```python
from build123d import *

# Parameters (mm, degrees)
SKETCH1_W           = 685.8
SKETCH1_H           = 165.1
BOSS_EXTRUDE1_DEPTH = 12.7
SKETCH2_R           = 3.175
CUT_EXTRUDE1_DEPTH  = 26.67
SKETCH3_R           = 3.5
CUT_EXTRUDE2_DEPTH  = 34
SKETCH4_R           = 6
CUT_EXTRUDE3_DEPTH  = 9.85
SKETCH5_R           = 1.7526
CUT_EXTRUDE4_DEPTH  = 19.05
SKETCH7_R           = 1.7526
CUT_EXTRUDE5_DEPTH  = 11.43


with BuildPart() as part:
    # Sketch1 → Boss-Extrude1 (new body)
    with BuildSketch(Plane.XY):
        Rectangle(SKETCH1_W, SKETCH1_H)
    extrude(amount=BOSS_EXTRUDE1_DEPTH)

    # Sketch2 → Cut-Extrude1 (cut)
    with BuildSketch(Plane(origin=(342.9, 0, 0), x_dir=(0, 0, -1), z_dir=(1, 0, 0))):
        with Locations((-6.35, -6.35)):
            Circle(SKETCH2_R)
    cut_extrude1 = extrude(amount=-CUT_EXTRUDE1_DEPTH, mode=Mode.SUBTRACT)

    # Sketch3 → Cut-Extrude2 (cut)
    with BuildSketch(Plane(origin=(342.9, 0, 0), x_dir=(0, 0, -1), z_dir=(1, 0, 0))):
        with Locations((-6.35, 38.1)):
            Circle(SKETCH3_R)
        with Locations(Location((-6.35, -50.8, 0), (0, 0, 180))):
            Circle(SKETCH3_R)
    cut_extrude2 = extrude(amount=-CUT_EXTRUDE2_DEPTH, mode=Mode.SUBTRACT)

    # Mirror2: Cut-Extrude1, Cut-Extrude2 across plane
    add(cut_extrude1.mirror(Plane(origin=(0, 0, 0), x_dir=(0, 0, 1), z_dir=(1, 0, 0))), mode=Mode.SUBTRACT)
    add(cut_extrude2.mirror(Plane(origin=(0, 0, 0), x_dir=(0, 0, 1), z_dir=(1, 0, 0))), mode=Mode.SUBTRACT)

    # Sketch4 → Cut-Extrude3 (cut)
    with BuildSketch(Plane.XY.offset(12.7)):
        with Locations((-308.9, 38.1)):
            Circle(SKETCH4_R)
        with Locations((308.9, -50.8)):
            Circle(SKETCH4_R)
        with Locations(Location((-308.9, -50.8, 0), (0, 0, 179.999999983))):
            Circle(SKETCH4_R)
        with Locations((308.9, 38.1)):
            Circle(SKETCH4_R)
    extrude(amount=-CUT_EXTRUDE3_DEPTH, mode=Mode.SUBTRACT)

    # Sketch5 → Cut-Extrude4 (cut)
    with BuildSketch(Plane.XZ.offset(82.55)):
        with Locations(Location((-209.55, 6.35, 0), (0, 0, 270))):
            Circle(SKETCH5_R)
        with Locations(Location((-69.85, 6.35, 0), (0, 0, 270))):
            Circle(SKETCH5_R)
        with Locations(Location((69.85, 6.35, 0), (0, 0, 270))):
            Circle(SKETCH5_R)
        with Locations(Location((209.55, 6.35, 0), (0, 0, 270))):
            Circle(SKETCH5_R)
    extrude(amount=-CUT_EXTRUDE4_DEPTH, mode=Mode.SUBTRACT)

    # Sketch7 → Cut-Extrude5 (cut)
    with BuildSketch(Plane(origin=(0, 0, 0), x_dir=(-1, 0, 0), z_dir=(0, 0, -1))):
        with Locations((278.43375, -61.9125)):
            Circle(SKETCH7_R)
        with Locations(Location((232.39625, -61.9125, 0), (0, 0, 180))):
            Circle(SKETCH7_R)
        with Locations((-232.39625, -61.9125)):
            Circle(SKETCH7_R)
        with Locations(Location((-278.43375, -61.9125, 0), (0, 0, 180))):
            Circle(SKETCH7_R)
    extrude(amount=-CUT_EXTRUDE5_DEPTH, mode=Mode.SUBTRACT)


solid = part.part
```
Could you check a few things on this model? Use its own coordinates, in mm. A direction names the side the tool comes from. Round coordinates to 2 decimals unless told otherwise and drop trailing zeros.
(1) Which directions (+Z, -Z, +X, -X, +Y, -Y) give clear straight access to the entire face, cutting with the end or side of a thin tool? Please do faces 1 (the face through (-309, -51, 2.85)), 2 (the face through (342.9, -1, 6)).
Findings below:
face 1: +Z
face 2: +Z, -Z, +X, +Y, -Y
(2) Thinking about a two-plate mould opening in Y: for faces 3 (the face through (-5, 82.55, 6)), 4 (the face through (302.906, 38.364, 7.844)), 5 (the face through (-5, -82.55, 6)), 6 (the face through (-5, 1, 0)), which applies, +Y half, -Y half, draft (parallel to the pull), parting line (faces both ways), or undercut?
Findings below:
face 3: +Y half
face 4: undercut
face 5: -Y half
face 6: draft
(3) If I drill on probe 1 along X at (y, z) = (-73, 6.35); probe 2 along Z at (x, y) = (336.5, 38.1); probe 3 along Z at (x, y) = (69, -67), over which ranges is the centre line in solid material (lowest first)?
Findings below:
probe 1: x = -342.9 to -211.3, -207.8 to -71.6, -68.1 to 68.1, 71.6 to 207.8, 211.3 to 342.9
probe 2: z = 0 to 2.85, 9.85 to 12.7
probe 3: z = 0 to 4.82, 7.88 to 12.7
(4) For pin 1 (2 mm diameter, centred on x = -271.5, y = 27.5, fed in from -Z); pin 2 (4 mm diameter, centred on y = 38.1, z = 6.35, fed in from +X); pin 3 (3 mm diameter, centred on y = -5.5, z = 7.5, fed in from -X); pin 4 (7 mm diameter, centred on x = -308.9, y = 38.1, fed in from +Z), each with a flat end and sliding along its axis, tell me the tip position at first contact or that it passes through.
Findings below:
pin 1: stops at z = 0
pin 2: stops at x = 303.24
pin 3: stops at x = -316.23
pin 4: stops at z = 2.85
